Autodesk Inventor part; units mm, degrees
ref_plane "YZ Plane" through (0, 0, 0) normal (1, 0, 0) x (0, 1, 0)
ref_plane "XZ Plane" through (0, 0, 0) normal (0, 1, 0) x (-1, 0, 0)
ref_plane "XY Plane" through (0, 0, 0) normal (0, 0, 1) x (1, 0, 0)
sketch "Sketch1" plane through (0, 0, 0) normal (0, 0, 1) x (1, 0, 0)
  line L0 (30, 0) -> (30, 5.439)
  line L1 (30, 5.439) -> (19.392, 5.439)
  line L2 (19.392, 5.439) -> (19.392, 2.5321)
  line L3 (12.155, 10.043) -> (0, 10.043)
  line L4 (0, 10.043) -> (0, 0)
  line L5 (0, 0) -> (30, 0)
  line L6 (12.155, 10.043) -> (12.155, 6.812)
  line L7 (12.155, 6.812) -> (19.392, 2.5321)
  dimension "d1" = 30
  dimension "d2" = 10.043
  dimension "d3" = 5.439
  dimension "d4" = 10.608
  dimension "d5" = 3.231
  dimension "d6" = 120.6
  dimension "d7" = 17.845
revolve "Revolution1" add sketch "Sketch1" angle 360 about axis through (0, 10.043, 0) along (0, -1, 0)
fillet "Fillet1" radius 1.5 1 edges at (-19.392, 2.5321, 0)
sketch "Sketch2" plane through (0, 0, 0) normal (0, -1, 0) x (1, 0, 0)
  circle A0 centre (0, 0) radius 30
  point P0 (25, 0)
  dimension "d10" = 25
hole "Hole1" at (25, 0, 0) direction (0, 1, 0) diameter 5 end through all
pattern_circular "Circular Pattern1" count 10 over 360 about axis through (0, -10, 0) along (0, 1, 0) of "Hole1"
sketch "Sketch3" plane through (0, 10.043, 0) normal (0, 1, 0) x (1, 0, 0)
  circle A0 centre (0, 0) radius 12.155
hole "Hole2" at (0, 10.043, 0) direction (0, -1, 0) diameter 7.936 end through all counterbore diameter 9.938 counterbore depth 7.672
sketch "Sketch4" plane through (0, 0, 0) normal (0, 0, 1) x (1, 0, 0)
  line L0 (-12.155, 10.043) -> (12.155, 10.043) construction
  line L1 (0, -6.974) -> (0, 27.06) construction
  point P0 (0, 10.043)
hole "Hole3" at (0, 10.043, 0) direction (0, 0, -1) diameter 6 end through all
properties part number "212-04" material "Steel, Alloy"
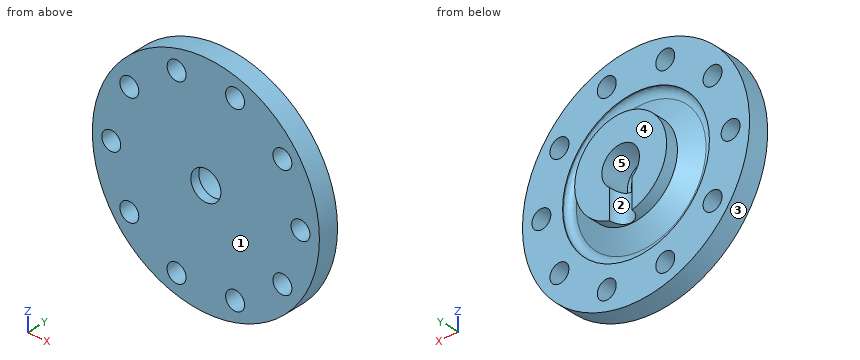
Could you check a few things on this model? Use its own coordinates, in mm. Face numbers are marked on the shaded views. A direction names the side the tool comes from. Give positions to 0.01 mm unless a question says otherwise; leave off trailing zeros. Order: outer loops, then holes, each group sorted by start corner. A loop starts at its lowest first (then second) coordinate and runs counter-clockwise, first axis right, second up. Notation, with made-up numbers: (46.25, -8.75) - (85.25, -8.75) arc R14 cw to (85.25, 9.25) - close; hole circle Ø6 at (48, 27.25). An arc over 180 degrees is marked (long way). One line per item, written item: value. Start each with the question number.
1. For the marked faces 4 and 5, which set-ups out of +Z, -Z, +X, -X, +Y, -Y let a thin tool reach every point of the face, with its end or its side?
2. For P1, Ø6.5, axis at x = -7.73, z = 23.78, coming from the +Y side; P2, Ø1, axis at y = 2.5, z = -1.5, coming from the +X side; P3, Ø3, axis at x = -17, y = 3.5, coming from the -Z side; P4, Ø4.5, axis at x = 7.73, z = 23.78, coming from the -Y side, each with a flat end and sliding along its axis, tell me the tip position at first contact or that it passes through.
3. Imagine slicing it at A-A on x = 25. List the corners of the cut face in (y, z) for me, plus the area to 3 significant figures.
4. Thinking about a two-plate mould opening in X: for the marked faces 1, 2 and 3, which applies, +X half, -X half, draft (parallel to the pull), parting line (faces both ways), or undercut?
5. If I drill on probe 1 along Z at (x, y) = (0, 0.6); probe 2 along Z at (x, y) = (8, 2.25); probe 3 along X at (y, z) = (3.75, -25.5), over which ranges is the centre line in solid material (lowest first)?
Values:
1. face 4: +Z, -Z, +X, -X, +Y
1. face 5: +Y
2. P1: y = 5.44
2. P2: x = 29.98
2. P3: z = -25.69
2. P4: through
3. outline: (0, -16.58) - (5.44, -16.58) - (5.44, -2.5) - (0, -2.5) - close; (0, 2.5) - (5.44, 2.5) - (5.44, 16.58) - (0, 16.58) - close
3. area: 153 mm²
4. face 1: draft
4. face 2: undercut
4. face 3: parting line
5. probe 1: -30 to -3.97, 3.97 to 30
5. probe 2: -28.91 to -26.26, -21.29 to 21.29, 26.26 to 28.91
5. probe 3: -15.8 to -9.54, -5.91 to 5.91, 9.54 to 15.8
